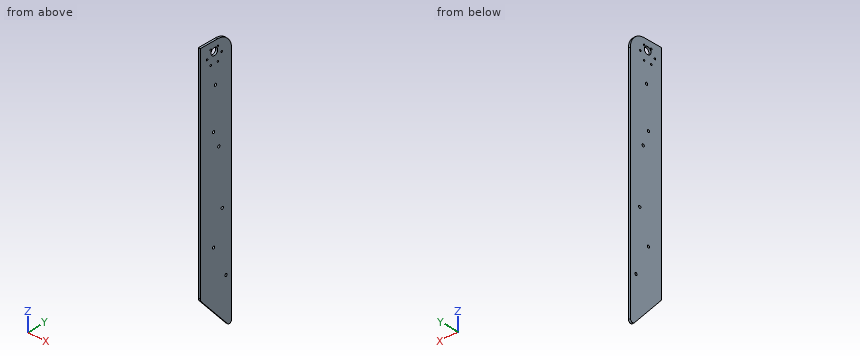
```python
from build123d import *

# Parameters (mm, degrees)
SKETCH_1_R      = 2.5
SKETCH_1_R_2    = 7
SKETCH_1_R_3    = 1.6
EXTRUDE_1_DEPTH = 4
FILLET_1_R      = 30


with BuildPart() as part:
    # 草图1 → 凸台-拉伸1 (new body)
    with BuildSketch(Plane.ZY):
        with BuildLine():
            Line((-206.943801285, -7), (226.406668198, -7))
            Line((226.406668198, -7), (226.406668198, 60))
            Line((226.406668198, 60), (-273.593331802, 60))
            ThreePointArc((-273.593331802, 60), (-278.27128826, 56.76542442), (-276.896763228, 51.246689353))
            Line((-276.896763228, 51.246689353), (-213.550664137, -4.506621294))
            ThreePointArc((-213.550664137, -4.506621294), (-210.474650125, -6.355912915), (-206.943801285, -7))
        make_face()
        with Locations((-191.007742204, 47.848052121)):
            Circle(SKETCH_1_R, mode=Mode.SUBTRACT)
        with Locations((68.992257796, 21.23337925)):
            Circle(SKETCH_1_R, mode=Mode.SUBTRACT)
        with Locations((38.992257796, 32.549891061)):
            Circle(SKETCH_1_R, mode=Mode.SUBTRACT)
        with Locations((-131.007742204, 21.23337925)):
            Circle(SKETCH_1_R, mode=Mode.SUBTRACT)
        with Locations((207.406668198, 23.006889262)):
            Circle(SKETCH_1_R_2, mode=Mode.SUBTRACT)
        with Locations((148.992257796, 25.23337925)):
            Circle(SKETCH_1_R, mode=Mode.SUBTRACT)
        with Locations((-71.007742204, 39.866402872)):
            Circle(SKETCH_1_R, mode=Mode.SUBTRACT)
        with Locations((213.830061956, 30.756889262)):
            Circle(SKETCH_1_R_3, mode=Mode.SUBTRACT)
        with Locations((200.406668198, 38.506889262)):
            Circle(SKETCH_1_R_3, mode=Mode.SUBTRACT)
        with Locations((186.983274439, 30.756889262)):
            Circle(SKETCH_1_R_3, mode=Mode.SUBTRACT)
        with Locations((186.983274439, 15.256889262)):
            Circle(SKETCH_1_R_3, mode=Mode.SUBTRACT)
        with Locations((200.406668198, 7.506889262)):
            Circle(SKETCH_1_R_3, mode=Mode.SUBTRACT)
        with Locations((213.830061956, 15.256889262)):
            Circle(SKETCH_1_R_3, mode=Mode.SUBTRACT)
    extrude(amount=EXTRUDE_1_DEPTH)

    # 圆角1
    fillet_1_edges = [part.edges().sort_by_distance(p)[0] for p in [
        (-2, 60, 226.406668198),
    ]]
    fillet(fillet_1_edges, radius=FILLET_1_R)


solid = part.part
```
Design review of the part built by this model. Coordinates are the model's own, in mm. Round coordinates to 2 decimals unless told otherwise and drop trailing zeros. Order: outer loops, then holes, each group sorted by start corner. A loop starts at its lowest first (then second) coordinate and runs counter-clockwise, first axis right, second up. Notation, with made-up numbers: (-26, 67.25) - (11, 67.25) arc R15 cw to (11, 80.25) - close; hole circle Ø2 at (-34.5, -6.75). An arc over 180 degrees is marked (long way). Return JSON: item names as keys, results as strings.
Q1. Consider section B-B on y = 0. Write out the cut boundary in (x, z), plus the area to 3 significant figures.
Computed values:
{"outline": "(-4, -218.67) - (0, -218.67) - (0, 226.41) - (-4, 226.41) - close", "area": "1,780 mm2"}
Q2. Consider section A-A on x = -1.6. Give the number of separate pieces and of enclosed holes in the cut face, plus the area to 3 significant figures.
Computed values:
{"separate pieces": "1", "enclosed holes": "13", "area": "31,300 mm2"}
Q3. Wall thickness on L1, parallel to Z at x = -2.35, y = 14; L2, parallel to Z at x = -3.2, y = 29.5; L3, parallel to Z at x = -0.2, y = 26.5: over which ranges is each line inside the solid? List them lowest first. Write a range as [from, to].
Computed values:
{"L1": "z = [-234.58, 185.99], [187.97, 212.84], [214.82, 226.41]", "L2": "z = [-252.19, 185.99], [187.97, 204.79], [210.02, 212.84], [214.82, 226.41]", "L3": "z = [-248.78, 146.84], [151.15, 201.34], [213.47, 226.41]"}
Q4. Consider section C-C on z = -227. Write out the cut boundary in (x, y).
Computed values:
{"outline": "(-4, 7.33) - (0, 7.33) - (0, 60) - (-4, 60) - close"}
